```python
from build123d import *

# Parameters (mm, degrees)
EXTRUDE_1_DEPTH     = 2
SKETCH_3_R          = 1.2
SKETCH_3_R_2        = 0.95
CUT_EXTRUDE_1_DEPTH = 2
SKETCH_4_W          = 56.3
SKETCH_4_H          = 2
EXTRUDE_2_DEPTH     = 13.8
SKETCH_5_R          = 1.2
SKETCH_5_R_2        = 0.95
SKETCH_5_W          = 13.8
SKETCH_5_H          = 5
SKETCH_5_H_2        = 2
EXTRUDE_3_DEPTH     = 2
SKETCH_6_W          = 43.55
SKETCH_6_H          = 2
CUT_EXTRUDE_2_DEPTH = 7.8
SKETCH_7_W          = 41.05
SKETCH_7_H          = 2
CUT_EXTRUDE_3_DEPTH = 3.9
EXTRUDE_4_DEPTH     = 13.8
SKETCH_9_W          = 25
SKETCH_9_H          = 3
EXTRUDE_5_DEPTH     = 56.3
SKETCH_10_W         = 33.55
SKETCH_10_H         = 56.3
SKETCH_10_H_2       = 2
EXTRUDE_6_DEPTH     = 2
SKETCH_11_W         = 56.3
SKETCH_11_H         = 2
CUT_EXTRUDE_4_DEPTH = 13.8
SKETCH_12_R         = 1.2
CUT_EXTRUDE_5_DEPTH = 166.991357908
SKETCH_16_R         = 1.2
CUT_EXTRUDE_6_DEPTH = 173.653387316
CHAMFER_1_SIZE      = 2
SKETCH_17_W         = 19
SKETCH_17_H         = 48.3
CUT_EXTRUDE_7_DEPTH = 10


with BuildPart() as part:
    # 草图2 → 凸台-拉伸1 (new body)
    with BuildSketch(Plane.XY):
        with BuildLine():
            Line((-24.5, 4.256503127), (-24.5, 20.182093825))
            Line((-24.5, 20.182093825), (-38.3, 20.182093825))
            Line((-38.3, 20.182093825), (-38.3, 12.382093825))
            Line((-38.3, 12.382093825), (-79.35, 12.382093825))
            Line((-79.35, 12.382093825), (-79.35, 20.182093825))
            Line((-79.35, 20.182093825), (-147.9, 20.182093825))
            Line((-147.9, 20.182093825), (-147.9, 1.662240991))
            Line((-147.9, 1.662240991), (-144.261, -4.817906175))
            Line((-144.261, -4.817906175), (-144.261, -14.817906175))
            Line((-144.261, -14.817906175), (-123.261, -14.817906175))
            Line((-123.261, -14.817906175), (-123.261, -3.217906175))
            ThreePointArc((-123.261, -3.217906175), (-117.3555, 2.687593825), (-111.45, -3.217906175))
            Line((-111.45, -3.217906175), (-111.45, -14.817906175))
            Line((-111.45, -14.817906175), (-34, -14.817906175))
            Line((-34, -14.817906175), (-34, -6.743496873))
            Line((-34, -6.743496873), (-24.5, 4.256503127))
        make_face()
    extrude(amount=-EXTRUDE_1_DEPTH)

    # 草图3 → 切除-拉伸1 (cut)
    with BuildSketch(Plane.XY):
        with Locations((-135.711, -8.917906175)):
            Circle(SKETCH_3_R)
        with Locations((-131.53, 1.032093825)):
            Circle(SKETCH_3_R_2)
        with Locations((-96.65, 1.032093825)):
            Circle(SKETCH_3_R_2)
        with BuildLine():
            ThreePointArc((-89.591805353, 1.032093825), (-89.296660471, 0.094597744), (-88.4, -0.307906175))
            ThreePointArc((-88.4, -0.307906175), (-87.551471863, 0.043565688), (-87.2, 0.892093825))
            ThreePointArc((-87.2, 0.892093825), (-87.202050413, 0.962213637), (-87.208194647, 1.032093825))
            Line((-87.208194647, 1.032093825), (-89.591805353, 1.032093825))
        make_face()
        with BuildLine():
            Line((-89.591805353, 1.032093825), (-87.208194647, 1.032093825))
            ThreePointArc((-87.208194647, 1.032093825), (-88.4, 2.092093825), (-89.591805353, 1.032093825))
        make_face()
        with BuildLine():
            ThreePointArc((-88.4, -10.207906175), (-87.551471863, -9.856434312), (-87.2, -9.007906175))
            ThreePointArc((-87.2, -9.007906175), (-87.551471863, -8.159378037), (-88.4, -7.807906175))
            Line((-88.4, -7.807906175), (-88.4, -10.207906175))
        make_face()
        with BuildLine():
            ThreePointArc((-88.4, -7.807906175), (-89.6, -9.007906175), (-88.4, -10.207906175))
            Line((-88.4, -10.207906175), (-88.4, -7.807906175))
        make_face()
        with BuildLine():
            ThreePointArc((-35.294856819, 1.032093825), (-35.136729236, -0.055043177), (-34.16, -0.557906175))
            ThreePointArc((-34.16, -0.557906175), (-33.311471863, -0.206434312), (-32.96, 0.642093825))
            ThreePointArc((-32.96, 0.642093825), (-32.976397832, 0.839795389), (-33.025143181, 1.032093825))
            Line((-33.025143181, 1.032093825), (-35.294856819, 1.032093825))
        make_face()
        with BuildLine():
            ThreePointArc((-33.025143181, 1.032093825), (-34.16, 1.842093825), (-35.294856819, 1.032093825))
            Line((-35.294856819, 1.032093825), (-33.025143181, 1.032093825))
        make_face()
        with BuildLine():
            ThreePointArc((-39.7, -9.007906175), (-39.348528137, -9.856434312), (-38.5, -10.207906175))
            ThreePointArc((-38.5, -10.207906175), (-37.651471863, -9.856434312), (-37.3, -9.007906175))
            Line((-37.3, -9.007906175), (-39.7, -9.007906175))
        make_face()
        with BuildLine():
            Line((-39.7, -9.007906175), (-37.3, -9.007906175))
            ThreePointArc((-37.3, -9.007906175), (-38.5, -7.807906175), (-39.7, -9.007906175))
        make_face()
    extrude(amount=-CUT_EXTRUDE_1_DEPTH, mode=Mode.SUBTRACT)

    # 草图4 → 凸台-拉伸2 (add)
    with BuildSketch(Plane.ZY.offset(38.3)):
        with Locations((-30.15, 14.182093825)):
            Rectangle(SKETCH_4_W, SKETCH_4_H)
    extrude(amount=-EXTRUDE_2_DEPTH)

    # 草图5 → 凸台-拉伸3 (add)
    # profile 1 of 3: a face of its own
    with BuildSketch(Plane(origin=(0, 0, -58.3), x_dir=(-1, 0, 0), z_dir=(0, 0, -1))):
        with BuildLine():
            ThreePointArc((123.261, -3.217906175), (117.3555, 2.687593825), (111.45, -3.217906175))
            Line((111.45, -3.217906175), (111.45, -14.817906175))
            Line((111.45, -14.817906175), (34, -14.817906175))
            Line((34, -14.817906175), (34, -6.743496873))
            Line((34, -6.743496873), (24.5, 4.256503127))
            Line((24.5, 4.256503127), (24.5, 13.182093825))
            Line((24.5, 13.182093825), (38.3, 13.182093825))
            Line((38.3, 13.182093825), (38.3, 12.382093825))
            Line((38.3, 12.382093825), (79.35, 12.382093825))
            Line((79.35, 12.382093825), (79.35, 20.182093825))
            Line((79.35, 20.182093825), (147.9, 20.182093825))
            Line((147.9, 20.182093825), (147.9, 1.662240991))
            Line((147.9, 1.662240991), (144.261, -4.817906175))
            Line((144.261, -4.817906175), (144.261, -14.817906175))
            Line((144.261, -14.817906175), (123.261, -14.817906175))
            Line((123.261, -14.817906175), (123.261, -3.217906175))
        make_face()
        with Locations(Location((135.711, -8.917906175, 0), (0, 0, 180))):
            Circle(SKETCH_5_R, mode=Mode.SUBTRACT)
        with Locations(Location((131.53, 1.032093825, 0), (0, 0, 180))):
            Circle(SKETCH_5_R_2, mode=Mode.SUBTRACT)
        with Locations(Location((96.65, 1.032093825, 0), (0, 0, 180))):
            Circle(SKETCH_5_R_2, mode=Mode.SUBTRACT)
        with Locations(Location((88.4, -9.007906175, 0), (0, 0, 180))):
            Circle(SKETCH_5_R, mode=Mode.SUBTRACT)
        with Locations(Location((88.4, 0.892093825, 0), (0, 0, 180))):
            Circle(SKETCH_5_R, mode=Mode.SUBTRACT)
        with Locations(Location((38.5, -9.007906175, 0), (0, 0, 180))):
            Circle(SKETCH_5_R, mode=Mode.SUBTRACT)
        with Locations(Location((34.16, 0.642093825, 0), (0, 0, 180))):
            Circle(SKETCH_5_R, mode=Mode.SUBTRACT)
    # profile 2 of 3: a face of its own
    with BuildSketch(Plane(origin=(0, 0, -58.3), x_dir=(-1, 0, 0), z_dir=(0, 0, -1))):
        with Locations((31.4, 17.682093825)):
            Rectangle(SKETCH_5_W, SKETCH_5_H)
    # profile 3 of 3: a face of its own
    with BuildSketch(Plane(origin=(0, 0, -58.3), x_dir=(-1, 0, 0), z_dir=(0, 0, -1))):
        with Locations((31.4, 14.182093825)):
            Rectangle(SKETCH_5_W, SKETCH_5_H_2)
    extrude(amount=EXTRUDE_3_DEPTH)

    # 草图6 → 切除-拉伸2 (cut)
    with BuildSketch(Plane(origin=(0, 20.182093825, 0), x_dir=(1, 0, 0), z_dir=(0, 1, 0))):
        with Locations((-126.125, 1)):
            Rectangle(SKETCH_6_W, SKETCH_6_H)
        with Locations((-126.125, 59.3)):
            Rectangle(SKETCH_6_W, SKETCH_6_H)
    extrude(amount=-CUT_EXTRUDE_2_DEPTH, mode=Mode.SUBTRACT)

    # 草图7 → 切除-拉伸3 (cut)
    with BuildSketch(Plane(origin=(0, 12.382093825, 0), x_dir=(1, 0, 0), z_dir=(0, 1, 0))):
        with Locations((-58.825, 1)):
            Rectangle(SKETCH_7_W, SKETCH_7_H)
        with Locations((-58.825, 59.3)):
            Rectangle(SKETCH_7_W, SKETCH_7_H)
    extrude(amount=-CUT_EXTRUDE_3_DEPTH, mode=Mode.SUBTRACT)

    # 草图8 → 凸台-拉伸4 (add)
    with BuildSketch(Plane.ZY.offset(38.3)):
        Polygon((-62.15, 25.182093825), (-60.3, 20.182093825), (-58.3, 20.182093825), (-58.3, 24.982093825), (-60.27, 24.982093825), (-60.27, 26.782093825), (-57.65, 26.782093825), (-57.65, 27.582093825), (-63.47, 27.582093825), (-63.47, 39.582093825), (-69.47, 39.582093825), (-69.47, 25.182093825), align=None)
        Polygon((-2, 24.982093825), (-2, 20.182093825), (0, 20.182093825), (1.85, 25.182093825), (10.33, 25.182093825), (10.33, 39.582093825), (4.33, 39.582093825), (4.33, 27.582093825), (-2.65, 27.582093825), (-2.65, 26.782093825), (-0.03, 26.782093825), (-0.03, 24.982093825), align=None)
    extrude(amount=-EXTRUDE_4_DEPTH)

    # 草图9 → 凸台-拉伸5 (add)
    with BuildSketch(Plane.XY.offset(-58.3)):
        with Locations((-91.85, 18.682093825)):
            Rectangle(SKETCH_9_W, SKETCH_9_H)
    extrude(amount=EXTRUDE_5_DEPTH)

    # 草图10 → 凸台-拉伸6 (add)
    with BuildSketch(Plane(origin=(0, 12.382093825, 0), x_dir=(1, 0, 0), z_dir=(0, 1, 0))):
        with Locations((-131.125, 30.15)):
            Rectangle(SKETCH_10_W, SKETCH_10_H)
        with Locations((-131.125, 1)):
            Rectangle(SKETCH_10_W, SKETCH_10_H_2)
        with Locations((-131.125, 59.3)):
            Rectangle(SKETCH_10_W, SKETCH_10_H_2)
    extrude(amount=EXTRUDE_6_DEPTH)

    # 草图11 → 切除-拉伸4 (cut)
    with BuildSketch(Plane.ZY.offset(38.3)):
        with Locations((-30.15, 14.182093825)):
            Rectangle(SKETCH_11_W, SKETCH_11_H)
    extrude(amount=-CUT_EXTRUDE_4_DEPTH, mode=Mode.SUBTRACT)

    # 草图12 → 切除-拉伸5 (cut, through all)
    with BuildSketch(Plane(origin=(0, 14.382093825, 0), x_dir=(1, 0, 0), z_dir=(0, 1, 0))):
        with Locations(Location((-117.55, 5.2, 0), (0, 0, 180))):
            Circle(SKETCH_12_R)
        with Locations(Location((-117.55, 55.1, 0), (0, 0, 180))):
            Circle(SKETCH_12_R)
        with Locations(Location((-144.7, 55.1, 0), (0, 0, 180))):
            Circle(SKETCH_12_R)
        with Locations(Location((-144.7, 5.2, 0), (0, 0, 180))):
            Circle(SKETCH_12_R)
    extrude(amount=-CUT_EXTRUDE_5_DEPTH, mode=Mode.SUBTRACT)

    # 草图16 → 切除-拉伸6 (cut, through all)
    with BuildSketch(Plane.XY.offset(10.33)):
        with Locations((-33.3, 32.732093825)):
            Circle(SKETCH_16_R)
    extrude(amount=-CUT_EXTRUDE_6_DEPTH, mode=Mode.SUBTRACT)

    # 倒角1
    chamfer_1_edges = [part.edges().sort_by_distance(p)[0] for p in [
        (-31.4, 25.182093825, -69.47),
        (-31.4, 25.182093825, 10.33),
    ]]
    chamfer(chamfer_1_edges, length=CHAMFER_1_SIZE)

    # 草图17 → 切除-拉伸7 (cut)
    with BuildSketch(Plane(origin=(0, 20.182093825, 0), x_dir=(1, 0, 0), z_dir=(0, 1, 0))):
        with Locations((-88.85, 30.15)):
            Rectangle(SKETCH_17_W, SKETCH_17_H)
    extrude(amount=-CUT_EXTRUDE_7_DEPTH, mode=Mode.SUBTRACT)


solid = part.part
```
Work out the finished part from the listing and answer in its coordinate system (mm). A direction names the side the tool comes from. Round coordinates to 2 decimals unless told otherwise and drop trailing zeros. Order: outer loops, then holes, each group sorted by start corner. A loop starts at its lowest first (then second) coordinate and runs counter-clockwise, first axis right, second up.
Q1. A tool of negligible diameter and unlimited length cuts with its end or side. For faces 1 (the flat face through (-100, 17.182, -31)), 2 (the flat face through (-38.3, 26, 4)), 3 (the flat face through (-31, 25.182, -65)), 4 (the flat face through (-98.35, 19, -30)), from which of +Z, -Z, +X, -X, +Y, -Y can it reach the whole face along a straight path? Write none if from no direction.
Solution:
face 1: +X, -X, -Y
face 2: +Z, -Z, +Y
face 3: -Z, +X, -X, -Y
face 4: +X, +Y, -Y
Q2. Given pin 1 Ø3.5 at (x, y) = (-86.5, 19) entering from +Z; pin 2 Ø1 at (y, z) = (-10, -59.5) entering from +X; pin 3 Ø1 at (x, z) = (-54, -1.5) entering from +Y, each flat-ended and moving along its own axis, determine where each tip first touches the part or whether it passes through.
Solution:
pin 1: stops at z = 0
pin 2: stops at x = -34
pin 3: stops at y = 8.48
Q3. Find the intervals of material crossed by line 1 along Z through (x, y) = (-117.55, 13.2); line 2 along Y through (x, z) = (-88.4, -59.2); line 3 along Y through (x, z) = (-34.16, -59.1), in increasing order.
Solution:
line 1: z = -60.3 to -56.3, -53.9 to -6.4, -4 to 0
line 2: y = -14.82 to -10.21, -7.81 to -0.31, 2.09 to 20.18
line 3: y = -14.82 to -0.56, 1.84 to 24.98, 26.78 to 27.58
Q4. The mould has two halves that part along X. Classify faces 5 (the cylindrical face through (-134.566, -8.557, -0.986)), 6 (the cylindrical face through (-116.35, 13.4, -5.15)), 7 (the flat face through (-29.3, -1.3, -1)), 8 (the flat face through (-31, 39.582, 7)): pulls with the +X half, pulls with the -X half, needs draft (parallel to the pull), parting line crosses it, or undercut.
Solution:
face 5: undercut
face 6: undercut
face 7: pulls with the +X half
face 8: needs draft
Q5. A cutting plane is placed at B-B, the plane x = -82. Determine the outline of the cut face in (y, z), then the cut area to 3 significant figures.
Solution:
outline: (-14.82, -60.3) - (20.18, -60.3) - (20.18, -54.3) - (17.18, -54.3) - (17.18, -58.3) - (-14.82, -58.3) - close; (-14.82, -2) - (17.18, -2) - (17.18, -6) - (20.18, -6) - (20.18, 0) - (-14.82, 0) - close
area: 164 mm2
Q6. A cutting plane is placed at A-A, the plane z = -46. Determine the outline of the cut face in (x, y), then the cut area to 3 significant figures.
Solution:
outline: (-147.9, 12.38) - (-114.35, 12.38) - (-114.35, 14.38) - (-147.9, 14.38) - close; (-104.35, 17.18) - (-98.35, 17.18) - (-98.35, 20.18) - (-104.35, 20.18) - close
area: 85.1 mm2
